Source: three-view drawing plus pictorial views. Frame: mm from the lowest corner of the part. A direction names the side the tool comes from. Give positions to 0.01 mm unless a question says otherwise; leave off trailing zeros. Order: outer loops, then holes, each group sorted by start corner. A loop starts at its lowest first (then second) coordinate and runs counter-clockwise, first axis right, second up. Notation, with made-up numbers: (89, -5.5) - (134, -5.5) arc R17 ccw to (134, 24.5) - close; hole circle Ø5 at (67, -28). An arc over 180 degrees is marked (long way). Use one line per item in the form item = value.
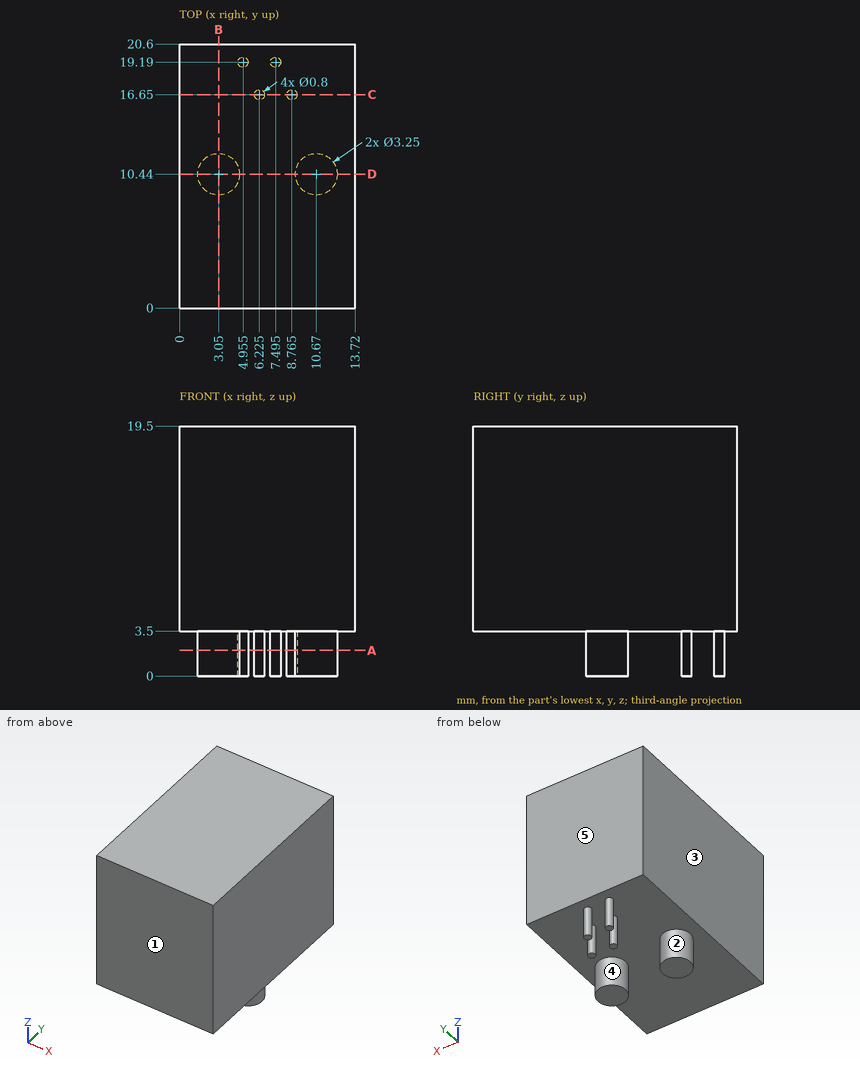
(1) Cut plane B-B on x = 3.05. Output: boundary loops of the cut face in (y, z) (3 decimals), plus the area to 3 significant figures.
Computed values:
outline = (0, 3.5) - (8.815, 3.5) - (8.815, 0) - (12.065, 0) - (12.065, 3.5) - (20.6, 3.5) - (20.6, 19.5) - (0, 19.5) - close
area = 341 mm²
(2) Ray query, line 1 along Z through (x, y) = (7, 10.5); line 2 along Y through (x, z) = (3.5, 2.5); line 3 along Y through (x, z) = (12, 2). Return the intervals inside material, ascending.
Computed values:
line_1 = 3.5 to 19.5
line_2 = 8.88 to 12
line_3 = 9.51 to 11.37
(3) Contact query for a flat-ended pin moving along its axis: pin 1 Ø2 at (x, y) = (5, 7.5) entering from -Z. Output: stop coordinate, or through.
Computed values:
pin_1 = 3.5
(4) Cut plane A-A on z = 2. Output: boundary loops of the cut face in (x, y) (3 decimals), plus the area to 3 significant figures.
Computed values:
outline = circle Ø3.25 at (3.05, 10.44); circle Ø0.8 at (4.955, 19.19); circle Ø0.8 at (6.225, 16.65); circle Ø0.8 at (7.495, 19.19); circle Ø0.8 at (8.765, 16.65); circle Ø3.25 at (10.67, 10.44)
area = 18.6 mm²
(5) Cut plane D-D on y = 10.44. Output: boundary loops of the cut face in (x, z) (3 decimals).
Computed values:
outline = (0, 3.5) - (1.425, 3.5) - (1.425, 0) - (4.675, 0) - (4.675, 3.5) - (9.045, 3.5) - (9.045, 0) - (12.295, 0) - (12.295, 3.5) - (13.72, 3.5) - (13.72, 19.5) - (0, 19.5) - close
(6) Pull-direction query (X, two-part tool) for the marked faces 3, 4 and 5; classes: released by +X, released by -X, zero draft, split by the parting line, or undercut.
Computed values:
face_3 = released by -X
face_4 = undercut
face_5 = zero draft
(7) Reachability of the marked faces 1 and 2 from +Z, -Z, +X, -X, +Y, -Y: full face, straight path, thin tool, end or side. Return the list, or none.
Computed values:
face_1 = +Z, -Z, +X, -X, -Y
face_2 = -Z
(8) Cut plane C-C on y = 16.65. Output: boundary loops of the cut face in (x, z) (3 decimals).
Computed values:
outline = (0, 3.5) - (5.825, 3.5) - (5.825, 0) - (6.625, 0) - (6.625, 3.5) - (8.365, 3.5) - (8.365, 0) - (9.165, 0) - (9.165, 3.5) - (13.72, 3.5) - (13.72, 19.5) - (0, 19.5) - close
